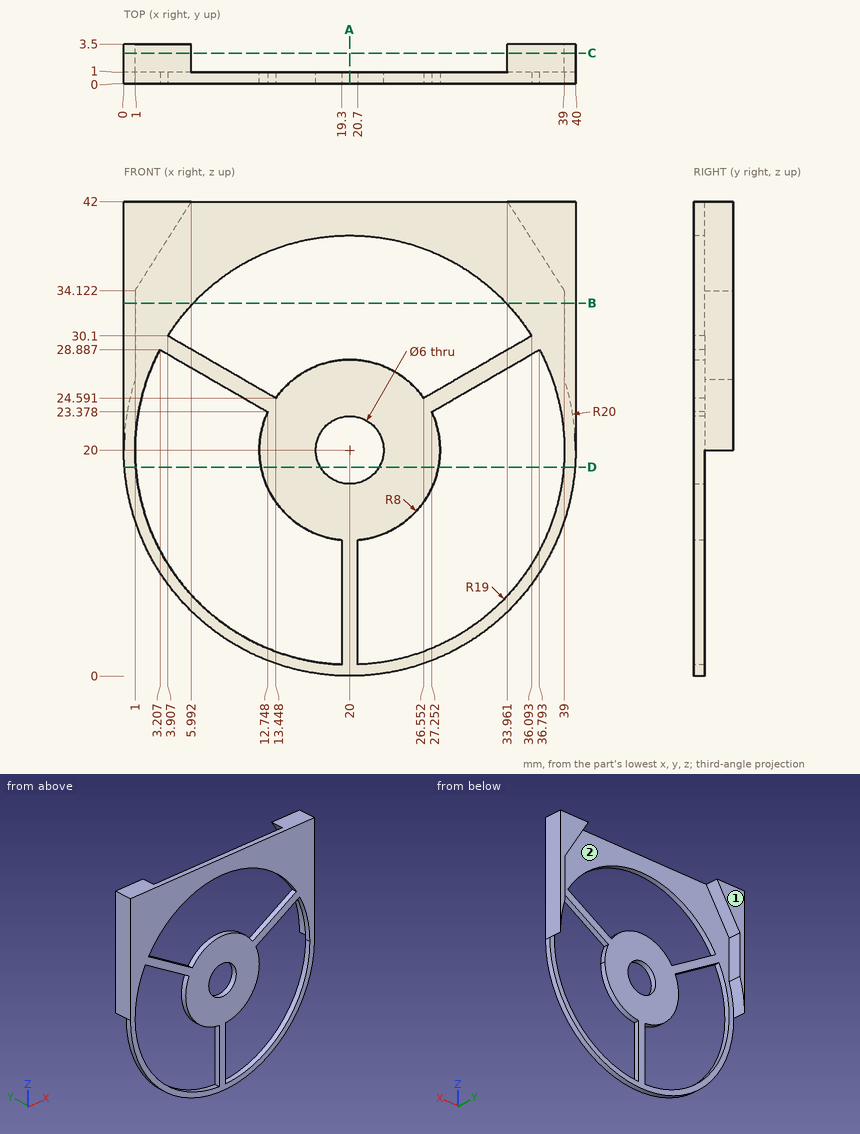
Drawing for the job (mm, zero at the part's lowest x, y, z). A direction names the side the tool comes from. Give positions to 0.01 mm unless a question says otherwise; leave off trailing zeros. Order: outer loops, then holes, each group sorted by start corner. A loop starts at its lowest first (then second) coordinate and runs counter-clockwise, first axis right, second up. Notation, with made-up numbers: (-6.75, 78.25) - (21.25, 78.25) arc R31 ccw to (21.25, 104.25) - close; hole circle Ø1 at (5, 88). An arc over 180 degrees is marked (long way). Write item = value, one per line. Start each with the question number.
1. Cut at D-D, the plane z = 18.5. List the corners of the cut face in (x, y).
2. Which spindle directions (+Z, -Z, +X, -X, +Y, -Y) get a long thin tool onto all of the face, cutting with end or side? Do the marked faces 1 and 2. Say none if no direction does.
3. Cut at A-A, the plane x = 20. List the corners of the cut face in (y, z).
4. Cut at B-B, the plane z = 33. List the corners of the cut face in (x, y).
5. Probe line 1 along X through (y, z) = (0.8, 20); line 2 along X through (y, z) = (0.7, 3.5) (1 decimal); line 3 along X through (y, z) = (2.05, 28.5). List the from-to ranges inside material, lowest first.
6. Cut at C-C, the plane y = 2.7. List the corners of the cut face in (x, z) (1 decimal).
7. Drop flat-ended pins along their axis: P1, Ø10, axis at x = 16, z = 5, coming from the -Y side; P2, Ø12, axis at x = 13, z = 17, coming from the +Y side; P3, Ø0.8, axis at y = 0.5, z = 7.5, coming from the +X side (1 decimal). Give the stop position or say it passes through.
Taken from the geometry:
q1.outline = (0.06, 0) - (1.06, 0) - (1.06, 1) - (0.06, 1) - close; (12.14, 0) - (17.4, 0) - (17.4, 1) - (12.14, 1) - close; (22.6, 0) - (27.86, 0) - (27.86, 1) - (22.6, 1) - close; (38.94, 0) - (39.94, 0) - (39.94, 1) - (38.94, 1) - close
q2.face_1 = +Z, -Z, +X, -X, +Y
q2.face_2 = -Z, +Y
q3.outline = (0, 0) - (1, 0) - (1, 17) - (0, 17) - close; (0, 23) - (1, 23) - (1, 28) - (0, 28) - close; (0, 39) - (1, 39) - (1, 42) - (0, 42) - close
q4.outline = (0, 0) - (6.14, 0) - (6.14, 1) - (1, 1) - (1, 3.5) - (0, 3.5) - close; (33.86, 0) - (40, 0) - (40, 3.5) - (39, 3.5) - (39, 1) - (33.86, 1) - close
q5.line_1 = 0 to 1, 12 to 17, 23 to 28, 39 to 40
q5.line_2 = 8.7 to 10.6, 19.3 to 20.7, 29.4 to 31.3
q5.line_3 = 0 to 1, 39 to 40
q6.outline = (0, 20) arc R20 cw to (1, 26.2) - (1, 34.1) - (6, 42) - (0, 42) - close; (34, 42) - (39, 34.1) - (39, 26.2) arc R20 cw to (40, 20) - (40, 42) - close
q7.P1 = 0
q7.P2 = 1
q7.P3 = 35.9
